```python
from build123d import *

# Parameters (mm, degrees)
SKETCH_1_R      = 1.5
EXTRUDE_1_DEPTH = 2
SKETCH_1_3_R    = 1.5
EXTRUDE_2_DEPTH = 4


with BuildPart() as part:
    # Sketch 1 → Extrude 1 (new body)
    with BuildSketch(Plane(origin=(0, 0, 0), x_dir=(1, 0, 0), z_dir=(0, 1, 0))):
        with BuildLine():
            Line((23.735839254, -5.318814311), (-23.735839254, -5.318814311))
            ThreePointArc((-23.735839254, -5.318814311), (-25.362389906, -4.839594543), (-26.469290407, -3.555036294))
            Line((-26.469290407, -3.555036294), (-34.277924852, 13.710892585))
            ThreePointArc((-34.277924852, 13.710892585), (-34.06525393, 16.57366522), (-31.544473698, 17.947114568))
            Line((-31.544473698, 17.947114568), (31.544473698, 17.947114568))
            ThreePointArc((31.544473698, 17.947114568), (34.06525393, 16.57366522), (34.277924852, 13.710892585))
            Line((34.277924852, 13.710892585), (26.469290407, -3.555036294))
            ThreePointArc((26.469290407, -3.555036294), (25.362389906, -4.839594543), (23.735839254, -5.318814311))
        make_face()
        with Locations(Location((-10.85, 11.75, 0), (0, 0, 270))):
            Circle(SKETCH_1_R, mode=Mode.SUBTRACT)
        with Locations(Location((10.85, 11.75, 0), (0, 0, 270))):
            Circle(SKETCH_1_R, mode=Mode.SUBTRACT)
    extrude(amount=EXTRUDE_1_DEPTH)

    # Sketch 1_3 → Extrude 2 (add)
    # profile 1 of 2: a face of its own
    with BuildSketch(Plane(origin=(0, 0, 0), x_dir=(1, 0, 0), z_dir=(0, 1, 0))):
        with BuildLine():
            Line((26.75, 16), (-26.75, 16))
            ThreePointArc((-26.75, 16), (-29.75520382, 14.75520382), (-31, 11.75))
            ThreePointArc((-31, 11.75), (-29.75520382, 8.74479618), (-26.75, 7.5))
            Line((-26.75, 7.5), (26.75, 7.5))
            ThreePointArc((26.75, 7.5), (31, 11.75), (26.75, 16))
        make_face()
        with Locations(Location((-10.85, 11.75, 0), (0, 0, 270))):
            Circle(SKETCH_1_3_R, mode=Mode.SUBTRACT)
        with Locations(Location((10.85, 11.75, 0), (0, 0, 270))):
            Circle(SKETCH_1_3_R, mode=Mode.SUBTRACT)
    # profile 2 of 2: a face of its own
    with BuildSketch(Plane(origin=(0, 0, 0), x_dir=(1, 0, 0), z_dir=(0, 1, 0))):
        with BuildLine():
            ThreePointArc((-25.671609734, 1.439529518), (-26.734805421, -0.212962113), (-25.25, -1.5))
            Line((-25.25, -1.5), (25.25, -1.5))
            ThreePointArc((25.25, -1.5), (26.734805421, -0.212962113), (25.671609734, 1.439529518))
            ThreePointArc((25.671609734, 1.439529518), (25.462962113, 1.484805421), (25.25, 1.5))
            Line((25.25, 1.5), (-25.25, 1.5))
            ThreePointArc((-25.25, 1.5), (-25.462962113, 1.484805421), (-25.671609734, 1.439529518))
        make_face()
    extrude(amount=EXTRUDE_2_DEPTH)


solid = part.part
```
Read the model definition and answer for the solid it produces. Units are mm, in the model's axes. A direction names the side the tool comes from. Give positions to 0.01 mm unless a question says otherwise; leave off trailing zeros. Order: outer loops, then holes, each group sorted by start corner. A loop starts at its lowest first (then second) coordinate and runs counter-clockwise, first axis right, second up. Notation, with made-up numbers: (11.25, 78) -> (62.25, 78) arc R24 ccw to (62.25, 105) -> close; hole circle Ø5 at (57.5, -21). An arc over 180 degrees is marked (long way). One line per item, written item: value. Start each with the question number.
(1) Straight lines are drawn through the part: L1, parallel to X at y = 2.8, z = -11.75; L2, parallel to Z at x = 15, y = 3.45; L3, parallel to X at y = 0.95, z = -11.75. For each, find the intervals that lie inside material, in ascending order.
(2) The part is cut by section D-D (z = -3.5). Determine the outline of the cut face in (x, y), and give its area (3 significant figures).
(3) A tool of negligible diameter and unlimited length cuts with its end or side. For faces 1 (the cylindrical face through (31, 3, -11.7)), 2 (the flat face through (0, 3, -1.5)), 3 (the flat face through (0, 3, 1.5)), 4 (the flat face through (0, 3, -16)), from which of +Z, -Z, +X, -X, +Y, -Y can it reach the whole face along a straight path? Write none if from no direction.
(4) The part is cut by section A-A (x = -10.85). Determine the outline of the cut face in (y, z), and give its area (3 significant figures).
(5) The part is cut by section B-B (y = 3.4). Determine the outline of the cut face in (x, z), and give its area (3 significant figures).
(6) Flat-ended cylindrical pins translate along their axes: P1, Ø1, axis at y = 1, z = -4.5, coming from the -X side; P2, Ø1.6, axis at x = 5.5, y = 3, coming from the -Z side. Find the tip coordinate at first contact, or state that the pin passes through.
(7) The part is cut by section C-C (x = 17). Determine the outline of the cut face in (y, z), and give its area (3 significant figures).
(8) For a pull along Z with two mould halves and no side action, classify faces 5 (the flat face through (0, 1, 5.319)), 6 (the cylindrical face through (-9.84, 1.97, -12.86)), 7 (the flat face through (0, 0, -6)) as released by +Z, released by -Z, zero draft, split by the parting line, or undercut.
Taken from the geometry:
1. L1: -31 to -12.35, -9.35 to 9.35, 12.35 to 31
1. L2: -16 to -7.5, -1.5 to 1.5
1. L3: -33.39 to -12.35, -9.35 to 9.35, 12.35 to 33.39
2. outline: (-29.66, 0) -> (29.66, 0) -> (29.66, 2) -> (-29.66, 2) -> close
2. area: 119 mm^2
3. face 1: +X, +Y
3. face 2: +X, -X, +Y
3. face 3: +Z, +X, -X, +Y
3. face 4: -Z, +X, -X, +Y
4. outline: (0, -17.95) -> (2, -17.95) -> (2, -16) -> (4, -16) -> (4, -13.25) -> (0, -13.25) -> close; (0, -10.25) -> (4, -10.25) -> (4, -7.5) -> (2, -7.5) -> (2, -1.5) -> (4, -1.5) -> (4, 1.5) -> (2, 1.5) -> (2, 5.32) -> (0, 5.32) -> close
4. area: 57.5 mm^2
5. outline: (-26.75, -16) -> (26.75, -16) arc R4.25 ccw to (26.75, -7.5) -> (-26.75, -7.5) arc R4.25 ccw to start; (-25.25, -1.5) -> (25.25, -1.5) arc R1.5 ccw to (25.25, 1.5) -> (-25.25, 1.5) arc R1.5 ccw to start; hole circle Ø3 at (-10.85, -11.75); hole circle Ø3 at (10.85, -11.75)
5. area: 656 mm^2
6. P1: x = -30.34
6. P2: z = -16
7. outline: (0, -17.95) -> (2, -17.95) -> (2, -16) -> (4, -16) -> (4, -7.5) -> (2, -7.5) -> (2, -1.5) -> (4, -1.5) -> (4, 1.5) -> (2, 1.5) -> (2, 5.32) -> (0, 5.32) -> close
7. area: 69.5 mm^2
8. face 5: released by +Z
8. face 6: undercut
8. face 7: zero draft
